The figure shows three views and two pictorial views of one solid part (mm, origin at its lowest corner). Answer the questions. Round coordinates to 2 decimals unless told otherwise and drop trailing zeros. Write each loop counter-clockwise with the first axis right and the second up, starting at its lowest first coordinate (ties: lowest second). Pieces come first, ordered by that corner, then holes. Notation, with made-up numbers: M 0.5,73.5 L 48.5,73.5 A6 ccw 48.5,77.5 Z; hole C 8.25,24.5 d6. An arc over 180 degrees is marked long. Answer in a Markdown table with one row per item.
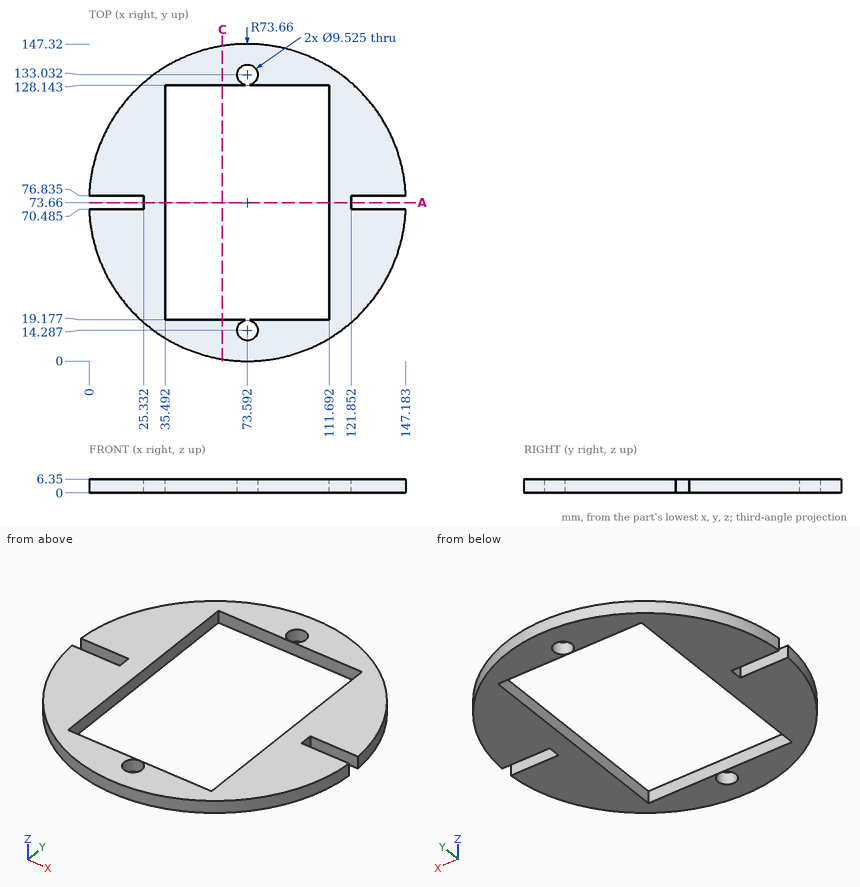
1. Consider line 1 along X through (y, z) = (74, 3.5); line 2 along Y through (x, z) = (15, 3.75) (1 decimal); line 3 along X through (y, z) = (58.5, 2) (1 decimal). Determine where each line is inside the solid, lowest interval first. Write a range as from..to.
Calculated:
| item | result |
|---|---|
| line 1 | x = 25.33..35.49, 111.69..121.85 |
| line 2 | y = 29..70.5, 76.8..118.3 |
| line 3 | x = 1.5..35.5, 111.7..145.7 |
2. Given pin 1 (1.9 mm diameter, centred on x = 8.5, z = 3.5, fed in from +Y) (1 decimal); pin 2 (1.9 mm diameter, centred on x = 77.5, z = 2.5, fed in from -Y); pin 3 (3 mm diameter, centred on y = 74.5, z = 3, fed in from +X), each flat-ended and moving along its own axis, determine where each tip first touches the part or whether it passes through.
Calculated:
| item | result |
|---|---|
| pin 1 | stops at y = 109.9 |
| pin 2 | stops at y = 0.06 |
| pin 3 | stops at x = 121.85 |
3. The part is cut by section C-C (x = 62). Determine the outline of the cut face in (y, z).
Calculated:
| item | result |
|---|---|
| outline | M 0.92,0 L 19.18,0 L 19.18,6.35 L 0.92,6.35 Z; M 128.14,0 L 146.4,0 L 146.4,6.35 L 128.14,6.35 Z |
4. The part is cut by section A-A (y = 73.66). Determine the outline of the cut face in (x, z), plus the area to 3 significant figures.
Calculated:
| item | result |
|---|---|
| outline | M 25.33,0 L 35.49,0 L 35.49,6.35 L 25.33,6.35 Z; M 111.69,0 L 121.85,0 L 121.85,6.35 L 111.69,6.35 Z |
| area | 129 mm² |
